Design review of the part built by this model. Coordinates are the model's own, in mm. A direction names the side the tool comes from. Coordinates: 2 decimals unless noted, no trailing zeros. Loops run counter-clockwise (first coordinate to the right, second up) from the corner with the lowest first, then second, coordinate; pieces in that order, holes last. Notation, with made-up numbers: (64, 11.25) - (87, 11.25) arc R18 ccw to (87, 16.25) - close; hole circle Ø9 at (41, 77.5). An arc over 180 degrees is marked (long way). Answer in a Markdown table with one row per item. Add a question column.
(1) We need section B-B, the plane z = 16.5. Give the number of separate pieces and of enclosed holes in the cut face, plus the area to 3 significant figures.
(2) The part is to be moulded in two halves that separate along X. For faces 5 (the face through (-2, -3.5, 15)), 6 (the face through (101.706, 26.521, 20.692)), 7 (the face through (3.61, 28.05, 14.79)), say which applies: released by +X, released by -X, zero draft, split by the parting line, or undercut.
(3) We need section A-A, the plane y = 55.5. Write out the cut boundary in (x, z).
(4) Clearance check with flat-ended pins moving along their axes: pin 1 (15 mm diameter, centred on y = 54.5, z = 19, fed in from -X); pin 2 (5 mm diameter, centred on y = 55.5, z = 8, fed in from +X); pin 3 (4 mm diameter, centred on y = 34.5, z = 26.5, fed in from -X); pin 4 (8 mm diameter, centred on x = 58, y = 49.5, fed in from -Z). State where each tip first meets the part, or that it passes through.
(5) We need section C-C, the plane x = 100. Write out the cut boundary in (y, z).
(6) To check wall thickness, follow L1, parallel to Z at x = 100, y = -2.3; L2, parallel to Y at x = 99, z = 19.5; L3, parallel to Z at x = 91, y = -4.5. State the ranges of each line that lie inside material, in increasing order. Write a range as [from, to].
(7) For faces 1 (the face through (0, -3, 15)), 2 (the face through (100, -0.5, 15)), 3 (the face through (-2, -6, 2.5)), 4 (the face through (97, -3.5, 15)), list the 3-axis set-ups (+Z, -Z, +X, -X, +Y, -Y) from which the entire face can be reached by the end or side of a thin tool; tool diameter is ignored.
(8) We need section D-D, the plane y = 38. Write out the cut boundary in (x, z).
from build123d import *

# Parameters (mm, degrees)
SKETCH1_W                = 5
SKETCH1_H                = 10
BOSS_EXTRUDE1_DEPTH      = 30
BOSS_EXTRUDE2_START      = -30
BOSS_EXTRUDE2_DEPTH      = 30
SKETCH3_W                = 25
SKETCH3_H                = 4
CUT_EXTRUDE1_DEPTH       = 121.665860955
BOSS_EXTRUDE3_REACH      = 122.666
BOSS_EXTRUDE3_END_RADIUS = 50
SKETCH4_W                = 30
SKETCH4_H                = 31.5
SKETCH5_W                = 30
SKETCH5_H                = 3
BOSS_EXTRUDE4_DEPTH      = 10
SKETCH6_R                = 2.15
CUT_EXTRUDE2_DEPTH       = 103.982097959
SKETCH7_R                = 2.15
CUT_EXTRUDE3_DEPTH       = 116.62439189


with BuildPart() as part:
    # Sketch1 → Boss-Extrude1 (new body)
    with BuildSketch(Plane.XY):
        with BuildLine():
            ThreePointArc((-5, 0), (45, 50), (95, 0))
            Line((95, 0), (90, 0))
            ThreePointArc((90, 0), (45, 45), (0, 0))
            Line((0, 0), (-5, 0))
        make_face()
        with Locations((92.5, -5)):
            Rectangle(SKETCH1_W, SKETCH1_H)
        with Locations((-2.5, -5)):
            Rectangle(SKETCH1_W, SKETCH1_H)
    extrude(amount=BOSS_EXTRUDE1_DEPTH)

    # Sketch2 → Boss-Extrude2 (add)
    with BuildSketch(Plane.XY.offset(30).offset(BOSS_EXTRUDE2_START)):
        with BuildLine():
            Line((32.25, 48.347052651), (32.25, 50))
            Line((32.25, 50), (32.25, 60.5))
            Line((32.25, 60.5), (27.25, 60.5))
            Line((27.25, 60.5), (27.25, 46.74331503))
            ThreePointArc((27.25, 46.74331503), (29.728932795, 47.610865424), (32.25, 48.347052651))
        make_face()
        with BuildLine():
            ThreePointArc((32.25, 48.347052651), (38.571649999, 49.585041255), (45, 50))
            Line((45, 50), (32.25, 50))
            Line((32.25, 50), (32.25, 48.347052651))
        make_face()
        with BuildLine():
            Line((32.25, 45), (45, 45))
            Line((45, 45), (45, 50))
            ThreePointArc((45, 50), (38.571649999, 49.585041255), (32.25, 48.347052651))
            Line((32.25, 48.347052651), (32.25, 45))
        make_face()
        with BuildLine():
            Line((45, 45), (57.75, 45))
            Line((57.75, 45), (57.75, 48.347052651))
            ThreePointArc((57.75, 48.347052651), (51.428350001, 49.585041255), (45, 50))
            Line((45, 50), (45, 45))
        make_face()
        with BuildLine():
            ThreePointArc((45, 50), (51.428350001, 49.585041255), (57.75, 48.347052651))
            Line((57.75, 48.347052651), (57.75, 50))
            Line((57.75, 50), (45, 50))
        make_face()
        with BuildLine():
            Line((57.75, 50), (57.75, 48.347052651))
            ThreePointArc((57.75, 48.347052651), (60.271067205, 47.610865424), (62.75, 46.74331503))
            Line((62.75, 46.74331503), (62.75, 60.5))
            Line((62.75, 60.5), (57.75, 60.5))
            Line((57.75, 60.5), (57.75, 50))
        make_face()
        with BuildLine():
            Line((27.25, 45), (32.25, 45))
            Line((32.25, 45), (32.25, 48.347052651))
            ThreePointArc((32.25, 48.347052651), (29.728932795, 47.610865424), (27.25, 46.74331503))
            Line((27.25, 46.74331503), (27.25, 45))
        make_face()
        with BuildLine():
            Line((57.75, 48.347052651), (57.75, 45))
            Line((57.75, 45), (62.75, 45))
            Line((62.75, 45), (62.75, 46.74331503))
            ThreePointArc((62.75, 46.74331503), (60.271067205, 47.610865424), (57.75, 48.347052651))
        make_face()
    extrude(amount=BOSS_EXTRUDE2_DEPTH)

    # Sketch3 → Cut-Extrude1 (cut, through all)
    with BuildSketch(Plane(origin=(95, 0, 0), x_dir=(0, 0, -1), z_dir=(1, 0, 0))):
        with Locations((-15, -5.5)):
            Rectangle(SKETCH3_W, SKETCH3_H)
    extrude(amount=-CUT_EXTRUDE1_DEPTH, mode=Mode.SUBTRACT)

    # Boss-Extrude3: up to this cylinder (the profile starts outside it)
    boss_extrude3_end = Plane(origin=(45, 0, 15), z_dir=(0, 0, -1)) * Cylinder(BOSS_EXTRUDE3_END_RADIUS, 346.332, mode=Mode.PRIVATE)
    # Sketch4 → Boss-Extrude3 (add, up to the surface)
    with BuildSketch(Plane(origin=(95, 0, 0), x_dir=(0, 0, -1), z_dir=(1, 0, 0)), mode=Mode.PRIVATE) as boss_extrude3_sk1:
        with Locations((-15, 12.25)):
            Rectangle(SKETCH4_W, SKETCH4_H)
    boss_extrude3_tool1 = extrude(boss_extrude3_sk1.sketch, amount=-BOSS_EXTRUDE3_REACH, mode=Mode.PRIVATE) - boss_extrude3_end
    add(boss_extrude3_tool1.solids().sort_by_distance((95, 12.25, 15))[0])
    add(boss_extrude3_tool1.solids().sort_by_distance((95, 12.25, 15))[1])

    # Sketch5 → Boss-Extrude4 (add)
    with BuildSketch(Plane(origin=(95, 0, 0), x_dir=(0, 0, -1), z_dir=(1, 0, 0))):
        with Locations((-15, -2)):
            Rectangle(SKETCH5_W, SKETCH5_H)
        with Locations((-15, 26.5)):
            Rectangle(SKETCH5_W, SKETCH5_H)
    extrude(amount=BOSS_EXTRUDE4_DEPTH)

    # Sketch6 → Cut-Extrude2 (cut, through all)
    with BuildSketch(Plane.ZY.offset(-27.25)):
        with Locations(Location((22, 55.5, 0), (0, 0, 180))):
            Circle(SKETCH6_R)
        with Locations(Location((8, 55.5, 0), (0, 0, 180))):
            Circle(SKETCH6_R)
    extrude(amount=-CUT_EXTRUDE2_DEPTH, mode=Mode.SUBTRACT)

    # Sketch7 → Cut-Extrude3 (cut, through all)
    with BuildSketch(Plane(origin=(0, 28, 0), x_dir=(1, 0, 0), z_dir=(0, 1, 0))):
        with Locations(Location((100, -22, 0), (0, 0, 180))):
            Circle(SKETCH7_R)
        with Locations(Location((100, -8, 0), (0, 0, 180))):
            Circle(SKETCH7_R)
    extrude(amount=-CUT_EXTRUDE3_DEPTH, mode=Mode.SUBTRACT)


solid = part.part
Responses:
| question | item | result |
|---|---|---|
| 1 | separate pieces | 3 |
| 1 | enclosed holes | 0 |
| 1 | area | 1,090 mm2 |
| 2 | face 5 | zero draft |
| 2 | face 6 | undercut |
| 2 | face 7 | released by -X |
| 3 | outline | (27.25, 0) - (32.25, 0) - (32.25, 5.85) - (27.25, 5.85) - close; (27.25, 10.15) - (32.25, 10.15) - (32.25, 19.85) - (27.25, 19.85) - close; (27.25, 24.15) - (32.25, 24.15) - (32.25, 30) - (27.25, 30) - close; (57.75, 0) - (62.75, 0) - (62.75, 5.85) - (57.75, 5.85) - close; (57.75, 10.15) - (62.75, 10.15) - (62.75, 19.85) - (57.75, 19.85) - close; (57.75, 24.15) - (62.75, 24.15) - (62.75, 30) - (57.75, 30) - close |
| 4 | pin 1 | stops at x = 27.25 |
| 4 | pin 2 | stops at x = 62.75 |
| 4 | pin 3 | stops at x = 7 |
| 4 | pin 4 | stops at z = 0 |
| 5 | outline | (-3.5, 0) - (-0.5, 0) - (-0.5, 5.85) - (-3.5, 5.85) - close; (-3.5, 10.15) - (-0.5, 10.15) - (-0.5, 19.85) - (-3.5, 19.85) - close; (-3.5, 24.15) - (-0.5, 24.15) - (-0.5, 30) - (-3.5, 30) - close; (25, 0) - (28, 0) - (28, 5.85) - (25, 5.85) - close; (25, 10.15) - (28, 10.15) - (28, 19.85) - (25, 19.85) - close; (25, 24.15) - (28, 24.15) - (28, 30) - (25, 30) - close |
| 6 | L1 | z = [0, 5.85], [10.15, 19.85], [24.15, 30] |
| 6 | L2 | y = [-3.5, -0.5], [25, 28] |
| 6 | L3 | z = [0, 2.5], [27.5, 30] |
| 7 | face 1 | +Z, -Z, -Y |
| 7 | face 2 | +Z, -Z, +X |
| 7 | face 3 | +X, -X |
| 7 | face 4 | +X |
| 8 | outline | (12.5, 0) - (20.9, 0) - (20.9, 30) - (12.5, 30) - close; (69.1, 0) - (77.5, 0) - (77.5, 30) - (69.1, 30) - close |
